```python
from build123d import *

# Parameters (mm, degrees)
F0_W     = 203.2
F0_H     = 50.8
F1_DEPTH = 19.05
F2_W     = 660.4
F2_H     = 12.699998945
F2_H_2   = 12.6999986589
F3_DEPTH = 6.35


# Not quite as in the source:
# - a feature names something its author has since deleted; it is built from what else it names


with BuildPart() as f1:
    # F0 (on Top) → F1 (new body)
    with BuildSketch(Plane.XY):
        Polygon((614.0642432213, 447.3863640726), (-46.3357567787, 447.3863640726), (-46.3357567787, -60.6136359274), (614.0642432213, -60.6136359274), (614.0642432213, -28.8636359274), (614.0642432213, -9.8136359274), (614.0642432213, 396.5863640726), (614.0642432213, 415.6363640726), align=None)
        with Locations((80.6642432213, 225.1363640726)):
            Rectangle(F0_W, F0_H, mode=Mode.SUBTRACT)
    extrude(amount=F1_DEPTH)

    # F2 (on face) → F3 (cut)
    with BuildSketch(Plane(origin=(0, 0, 0), x_dir=(1, 0, 0), z_dir=(0, 0, -1))):
        with Locations((283.8642432213, -282.2863646001)):
            Rectangle(F2_W, F2_H)
        with Locations((283.8642432213, -104.4863647431)):
            Rectangle(F2_W, F2_H_2)
    extrude(amount=-F3_DEPTH, mode=Mode.SUBTRACT)


solid = f1.part
```
The listing builds one solid part. Answer for the finished solid, in the listing's coordinates (mm). A direction names the side the tool comes from. Coordinates: 2 decimals unless noted, no trailing zeros. Loops run counter-clockwise (first coordinate to the right, second up) from the corner with the lowest first, then second, coordinate; pieces in that order, holes last. Notation, with made-up numbers: (51, 74) - (88, 74) arc R35 cw to (88, 109) - close; hole circle Ø10 at (-31, 1.5). An arc over 180 degrees is marked (long way). Use a Markdown table: item, result. Add a question column.
1) Find the intervals of material crossed by line 1 (Y direction, x = 228.5, z = 2.75); line 2 (Y direction, x = 142.5, z = 5.5); line 3 (Y direction, x = 133, z = 7.5), in increasing order.
2) The mould has two halves that part along Y. Classify faces 4 (the flat face through (279, 197, 19.05)), 5 (the flat face through (279, -60.614, 9)), 6 (the flat face through (79, 250.536, 9)): released by +Y, released by -Y, zero draft, split by the parting line, or undercut.
3) For faces 1 (the flat face through (79, 199.736, 9)), 2 (the flat face through (279, 369, 0)), 3 (the flat face through (279, 104, 6.35)), determine the directions among +Z, -Z, +X, -X, +Y, -Y from which every point of the face is accessible in a straight line to the end or side of a thin tool.
4) The part is cut by section C-C, the plane x = 173. Give the vertices of the cut face in (y, z).
5) The part is cut by section A-A, the plane z = 13.25. Give the vertices of the cut face in (x, y), and give its area (3 significant figures).
6) The part is cut by section B-B, the plane y = 233.5. Give the vertices of the cut face in (x, z), and give its area (3 significant figures).
7) Given pin 1 (10 mm diameter, centred on x = 307, y = 105.5, fed in from -Z), flat-ended and moving along its own axis, determine where the tip first touches the part or whether it passes through.
8) The part is cut by section D-D, the plane x = 336.5. Give the vertices of the cut face in (y, z), and give its area (3 significant figures).
Here are the results:
| question | item | result |
|---|---|---|
| 1 | line 1 | y = -60.61 to 98.14, 110.84 to 275.94, 288.64 to 447.39 |
| 1 | line 2 | y = -60.61 to 98.14, 110.84 to 199.74, 250.54 to 275.94, 288.64 to 447.39 |
| 1 | line 3 | y = -60.61 to 199.74, 250.54 to 447.39 |
| 2 | face 4 | zero draft |
| 2 | face 5 | released by -Y |
| 2 | face 6 | undercut |
| 3 | face 1 | +Z, -Z |
| 3 | face 2 | -Z, +X, -X, +Y, -Y |
| 3 | face 3 | -Z, +X, -X |
| 4 | outline | (-60.61, 0) - (98.14, 0) - (98.14, 6.35) - (110.84, 6.35) - (110.84, 0) - (199.74, 0) - (199.74, 19.05) - (-60.61, 19.05) - close; (250.54, 0) - (275.94, 0) - (275.94, 6.35) - (288.64, 6.35) - (288.64, 0) - (447.39, 0) - (447.39, 19.05) - (250.54, 19.05) - close |
| 5 | outline | (-46.34, -60.61) - (614.06, -60.61) - (614.06, 447.39) - (-46.34, 447.39) - close; hole (-20.94, 199.74) - (182.26, 199.74) - (182.26, 250.54) - (-20.94, 250.54) - close |
| 5 | area | 325,000 mm^2 |
| 6 | outline | (-46.34, 0) - (-20.94, 0) - (-20.94, 19.05) - (-46.34, 19.05) - close; (182.26, 0) - (614.06, 0) - (614.06, 19.05) - (182.26, 19.05) - close |
| 6 | area | 8,710 mm^2 |
| 7 | pin 1 | stops at z = 6.35 |
| 8 | outline | (-60.61, 0) - (98.14, 0) - (98.14, 6.35) - (110.84, 6.35) - (110.84, 0) - (275.94, 0) - (275.94, 6.35) - (288.64, 6.35) - (288.64, 0) - (447.39, 0) - (447.39, 19.05) - (-60.61, 19.05) - close |
| 8 | area | 9,520 mm^2 |
